from build123d import *

# Parameters (mm, degrees)
EXTRUDE1_DEPTH                                       = 88.9
EXTRUDE2_DEPTH                                       = 12.7
EXTRUDE3_DEPTH                                       = 3.175
CBORE_FOR_1_4_BINDING_HEAD_MACHINE_SCREW_D           = 9.525
CBORE_FOR_1_4_BINDING_HEAD_MACHINE_SCREW_CBORE_D     = 17.4752
CBORE_FOR_1_4_BINDING_HEAD_MACHINE_SCREW_CBORE_DEPTH = 3.175
F_1_4_20_TAPPED_HOLE1_AT_2_COUNT                     = 2
F_1_4_20_TAPPED_HOLE1_AT_2_PITCH                     = 50.8
FILLET2_R                                            = 3.175
FILLET2_OF_MIRROR1_R                                 = 3.175


with BuildPart() as part:
    # Sketch1 → Extrude1 (new body)
    with BuildSketch(Plane.XY):
        with BuildLine():
            Line((69.85, 25.4), (123.825, 25.4))
            Line((123.825, 25.4), (123.825, 15.875))
            ThreePointArc((123.825, 15.875), (124.75493597, 13.62993597), (127, 12.7))
            Line((127, 12.7), (139.7, 12.7))
            Line((139.7, 12.7), (139.7, 0))
            Line((139.7, 0), (101.6, 0))
            Line((101.6, 0), (101.6, 1.5748))
            ThreePointArc((101.6, 1.5748), (100.201376302, 4.951376302), (96.8248, 6.35))
            Line((96.8248, 6.35), (69.85, 6.35))
            Line((69.85, 6.35), (69.85, 25.4))
        make_face()
    extrude1 = extrude(amount=-EXTRUDE1_DEPTH)

    # Sketch2 → Extrude2 (add)
    with BuildSketch(Plane(origin=(0, 0, 0), x_dir=(1, 0, 0), z_dir=(0, 1, 0))):
        with BuildLine():
            Line((139.7, 57.15), (139.7, 88.9))
            ThreePointArc((139.7, 88.9), (155.575, 73.025), (139.7, 57.15))
        make_face()
        with BuildLine():
            Line((139.7, 31.75), (139.7, 0))
            ThreePointArc((139.7, 0), (155.575, 15.875), (139.7, 31.75))
        make_face()
    extrude2 = extrude(amount=EXTRUDE2_DEPTH)

    # Sketch3 → Extrude3 (cut)
    with BuildSketch(Plane(origin=(123.825, 25.4, 0), x_dir=(-1, 0, 0), z_dir=(0, 1, 0))):
        with BuildLine():
            Line((0, -82.55), (25.4, -82.55))
            ThreePointArc((25.4, -82.55), (29.890128061, -80.690128061), (31.75, -76.2))
            Line((31.75, -76.2), (31.75, -12.7))
            ThreePointArc((31.75, -12.7), (29.890128061, -8.209871939), (25.4, -6.35))
            Line((25.4, -6.35), (0, -6.35))
            Line((0, -6.35), (0, -82.55))
        make_face()
    extrude3 = extrude(amount=-EXTRUDE3_DEPTH, mode=Mode.SUBTRACT)

    # CBORE for 1/4 Binding Head Machine Screw1 (through all)
    with Locations(Plane(origin=(139.7, 12.7, -73.025), x_dir=(0, 0, 1), z_dir=(0, 1, 0))):
        with Locations((0, 0), (57.15, 0)):
            cbore_for_1_4_binding_head_machine_screw = CounterBoreHole(CBORE_FOR_1_4_BINDING_HEAD_MACHINE_SCREW_D / 2, CBORE_FOR_1_4_BINDING_HEAD_MACHINE_SCREW_CBORE_D / 2, CBORE_FOR_1_4_BINDING_HEAD_MACHINE_SCREW_CBORE_DEPTH)

    # Sketch5 → 1/4-20 Tapped Hole1 (revolve, cut)
    with BuildSketch(Plane(origin=(111.125, 22.225, -19.05), x_dir=(0, 0, 1), z_dir=(1, 0, 0))):
        Polygon((0, 0), (0, 17.535816902), (2.5527, 16.002), (2.5527, 12.7), (3.175, 12.7), (3.175, 0), align=None)
    f_1_4_20_tapped_hole1 = revolve(axis=Axis((111.125, 28.575, -19.05), (0, -1, 0)), mode=Mode.SUBTRACT)

    # 1/4-20 Tapped Hole1 at 2: 1/4-20 Tapped Hole1 ×2
    with Locations(*[(0, 0, -i * F_1_4_20_TAPPED_HOLE1_AT_2_PITCH) for i in range(1, F_1_4_20_TAPPED_HOLE1_AT_2_COUNT)]):
        add(f_1_4_20_tapped_hole1, mode=Mode.SUBTRACT)

    # Fillet2
    fillet2_edges = [part.edges().sort_by_distance(p)[0] for p in [
        (139.7, 6.35, -57.15),
        (139.7, 6.35, -31.75),
    ]]
    fillet(fillet2_edges, radius=FILLET2_R)

    # Mirror1: Extrude1, Extrude2, Extrude3, CBORE for 1/4 Binding Head Machine Screw1, 1/4-20 Tapped Hole1 across plane
    add(extrude1.mirror(Plane(origin=(69.85, 25.4, -88.9), x_dir=(0, 0, 1), z_dir=(-1, 0, 0))))
    add(extrude2.mirror(Plane(origin=(69.85, 25.4, -88.9), x_dir=(0, 0, 1), z_dir=(-1, 0, 0))))
    add(extrude3.mirror(Plane(origin=(69.85, 25.4, -88.9), x_dir=(0, 0, 1), z_dir=(-1, 0, 0))), mode=Mode.SUBTRACT)
    add(cbore_for_1_4_binding_head_machine_screw.mirror(Plane(origin=(69.85, 25.4, -88.9), x_dir=(0, 0, 1), z_dir=(-1, 0, 0))), mode=Mode.SUBTRACT)
    add(f_1_4_20_tapped_hole1.mirror(Plane(origin=(69.85, 25.4, -88.9), x_dir=(0, 0, 1), z_dir=(-1, 0, 0))), mode=Mode.SUBTRACT)

    # Mirror1 copy 1 sketch → Mirror1 copy 1 (revolve, cut)
    with BuildSketch(Plane(origin=(28.575, 22.225, -69.85), x_dir=(0, 0, 1), z_dir=(-1, 0, 0))):
        Polygon((0, 0), (0, -17.535816902), (2.5527, -16.002), (2.5527, -12.7), (3.175, -12.7), (3.175, 0), align=None)
    revolve(axis=Axis((28.575, 28.575, -69.85), (0, 1, 0)), mode=Mode.SUBTRACT)

    # Fillet2 of Mirror1
    fillet2_of_mirror1_edges = [part.edges().sort_by_distance(p)[0] for p in [
        (0, 6.35, -57.15),
        (0, 6.35, -31.75),
    ]]
    fillet(fillet2_of_mirror1_edges, radius=FILLET2_OF_MIRROR1_R)


solid = part.part
Geometry: final body of the model. Coordinates: model frame, mm. A direction names the side the tool comes from. Give positions to 0.01 mm unless a question says otherwise; leave off trailing zeros. Order: outer loops, then holes, each group sorted by start corner. A loop starts at its lowest first (then second) coordinate and runs counter-clockwise, first axis right, second up. Notation, with made-up numbers: (-23.75, 72) -> (25.25, 72) arc R34 cw to (25.25, 105) -> close; hole circle Ø10 at (51, 36.5). An arc over 180 degrees is marked (long way). Put each result on its own line as item: value.
Q1. Material intervals for L1, parallel to Z at x = 25.5, y = 23.5; L2, parallel to Y at x = 17, z = -53.5 (3 decimals); L3, parallel to Y at x = 65.5, z = -13.5, sorted ascending.
Here are the results:
L1: z = -88.9 to -82.55, -6.35 to 0
L2: y = 0 to 22.225
L3: y = 6.35 to 25.4
Q2. Reachability of faces 1 (the face through (111, 24, -6.35)), 2 (the face through (29, 24, -6.35)), 3 (the face through (136, 9.525, -69)), 4 (the face through (-0.77, 6.439, -56.315)) from +Z, -Z, +X, -X, +Y, -Y: full face, straight path, thin tool, end or side. Return the list, or none.
Here are the results:
face 1: +X, +Y
face 2: -X, +Y
face 3: +Y
face 4: -X, +Y, -Y
Q3. Section D-D, the plane x = 64. Return loops of the section in (y, z), then the cut area to 3 significant figures.
Here are the results:
outline: (6.35, -88.9) -> (25.4, -88.9) -> (25.4, 0) -> (6.35, 0) -> close
area: 1,690 mm^2
Q4. Section B-B, the plane z = -26.5. Return loops of the section in (x, y) (3 decimals).
Here are the results:
outline: (-11.795, 0) -> (38.1, 0) -> (38.1, 1.575) arc R4.775 cw to (42.875, 6.35) -> (96.825, 6.35) arc R4.775 cw to (101.6, 1.575) -> (101.6, 0) -> (151.495, 0) -> (151.495, 12.7) -> (127, 12.7) arc R3.175 cw to (123.825, 15.875) -> (123.825, 22.225) -> (92.075, 22.225) -> (92.075, 25.4) -> (47.625, 25.4) -> (47.625, 22.225) -> (15.875, 22.225) -> (15.875, 15.875) arc R3.175 cw to (12.7, 12.7) -> (-11.795, 12.7) -> close
Q5. Section A-A, the plane x = 23. Return loops of the section in (y, z) (3 decimals), then the cut area to 3 significant figures.
Here are the results:
outline: (0, -88.9) -> (25.4, -88.9) -> (25.4, -82.55) -> (22.225, -82.55) -> (22.225, -6.35) -> (25.4, -6.35) -> (25.4, 0) -> (0, 0) -> close
area: 2,020 mm^2
Q6. Pin query (flat end, axial travel): pin 1 (8 mm diameter, centred on y = 20.5, z = -64.5, fed in from +X) (3 decimals); pin 2 (16 mm diameter, centred on x = 31, z = -37, fed in from +Y) (3 decimals); pin 3 (3 mm diameter, centred on x = 36, y = 12.5, fed in from +Z); pin 4 (14 mm diameter, centred on x = 139, z = -75.5, fed in from +Y). Return the tip coordinate at first contact, or that it passes through.
Here are the results:
pin 1: stops at x = 123.825
pin 2: stops at y = 22.225
pin 3: stops at z = 0
pin 4: stops at y = 12.7
Q7. Draft query along X for faces 5 (the face through (69, 13, 0)), 6 (the face through (114, 9.525, -70)), 7 (the face through (47.625, 24, -45)). Return one class per face: released by +X, released by -X, zero draft, split by the parting line, or undercut.
Here are the results:
face 5: zero draft
face 6: undercut
face 7: released by -X
Q8. Section C-C, the plane x = 45.5. Return loops of the section in (y, z) (3 decimals).
Here are the results:
outline: (6.35, -88.9) -> (25.4, -88.9) -> (25.4, -80.94) -> (22.225, -80.94) -> (22.225, -7.96) -> (25.4, -7.96) -> (25.4, 0) -> (6.35, 0) -> close
